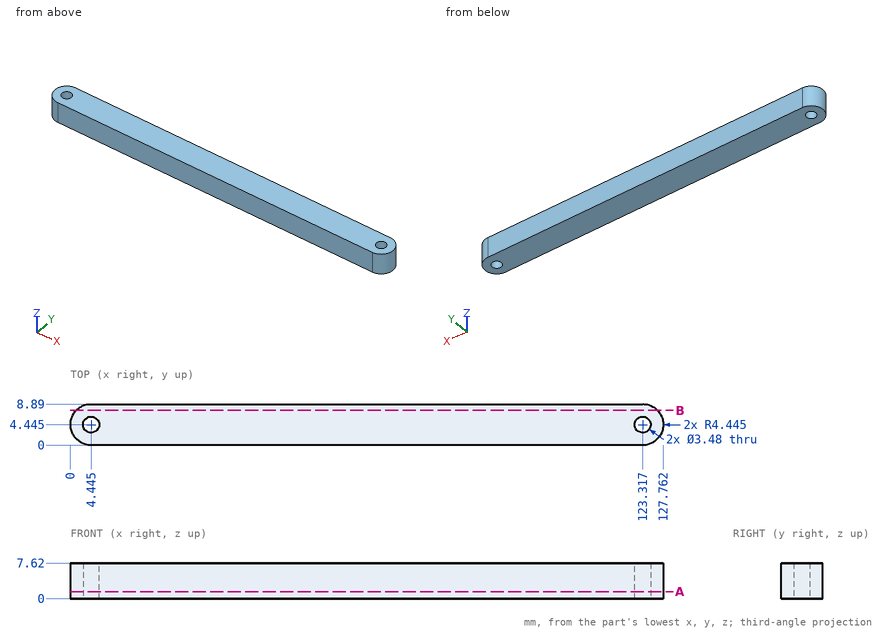
Check sheet for the drawn part. Datum: minimum x, y, z corner. Units: mm. Round coordinates to 2 decimals unless told otherwise and drop trailing zeros. Order: outer loops, then holes, each group sorted by start corner. A loop starts at its lowest first (then second) coordinate and runs counter-clockwise, first axis right, second up. Notation, with made-up numbers: M 20.25,-32.5 L 60.25,-32.5 A23 ccw 60.25,-13.5 Z; hole C 47,7.5 d2. An arc over 180 degrees is marked long. Write each question's results on one line, items separated by ' | '. Start each with the question number.
1. Cross-section at B-B on y = 7.5. Record the boundary of the cut face in (x, z).
2. Cross-section at A-A on z = 1.5. Record the boundary of the cut face in (x, y) (1 decimal), plus the area to 3 significant figures.
3. Go/stop test with flat-tipped pins: P1, Ø1.5, axis at y = 2, z = 5, coming from the -X side; P2, Ø4, axis at y = 1, z = 1, coming from the -X side; P3, Ø2, axis at y = 3, z = 2, coming from the +X side. Record where each tip stops, or that it passes through.
4. Material ranges on L1, parallel to X at y = 4.5, z = 6.75; L2, parallel to X at y = 3.25, z = 0.75; L3, parallel to Y at x = 122.5, z = 4.75, recorded low to high. Write a range as from..to.
Resolved:
1) outline: M 1.22,0 L 126.55,0 L 126.55,7.62 L 1.22,7.62 Z
2) outline: M 4.4,0 L 123.3,0 A4.4 ccw 123.3,8.9 L 4.4,8.9 A4.4 ccw Z; hole C 4.4,4.4 d3.5; hole C 123.3,4.4 d3.5 | area: 1,100 mm2
3) P1: x = 0.34 | P2: x = 0.24 | P3: x = 127.74
4) L1: 0..2.71, 6.18..121.58, 125.06..127.76 | L2: 0.16..3.18, 5.71..122.05, 124.58..127.6 | L3: 0..2.91, 5.98..8.89
